Verification items for this drawing (mm, ordinates from the low corner). A direction names the side the tool comes from. Round coordinates to 2 decimals unless told otherwise and drop trailing zeros. Loops run counter-clockwise (first coordinate to the right, second up) from the corner with the lowest first, then second, coordinate; pieces in that order, holes last. Notation, with made-up numbers: M 73,-24 L 87,-24 A21 ccw 87,-20 Z; hole C 41.25,30.25 d10. An arc over 180 degrees is marked long. One line per item, written item: value.
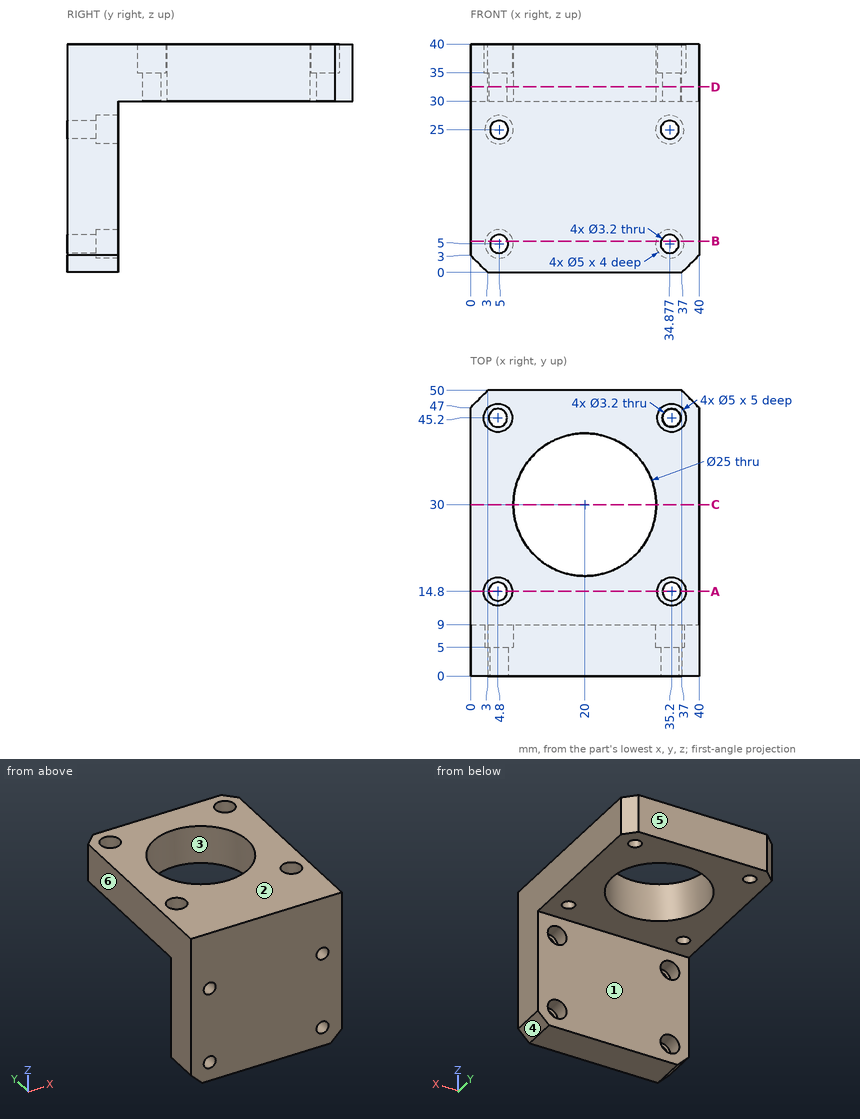
(1) Tool access check on the marked faces 1 and 2. Record the directions out of +Z, -Z, +X, -X, +Y, -Y that give a thin tool (end or side, any length) a straight path to the whole face; none if there is none.
Completed:
face 1: -Z, +X, -X, +Y
face 2: +Z, +X, -X, +Y, -Y
(2) Mould release check, pull along X, two halves, no side actions. Record for the marked faces 3, 4, 5 and 6: +X half, -X half, draft (parallel to the pull), parting line (faces both ways), or undercut.
Completed:
face 3: undercut
face 4: +X half
face 5: draft
face 6: -X half
(3) Sectioned sample at A-A on y = 14.8. Enter the section's corners in (x, z).
Completed:
outline: M 0,30 L 3.2,30 L 3.2,35 L 2.3,35 L 2.3,40 L 0,40 Z; M 6.4,30 L 33.6,30 L 33.6,35 L 32.7,35 L 32.7,40 L 7.3,40 L 7.3,35 L 6.4,35 Z; M 36.8,30 L 40,30 L 40,40 L 37.7,40 L 37.7,35 L 36.8,35 Z
(4) Depth check by flat-ended pin: pin 1 Ø2.5 at (x, z) = (34, 5.5) entering from +Y; pin 2 Ø6 at (x, y) = (33.5, 44) entering from -Z; pin 3 Ø1.9 at (x, y) = (35.2, 45.2) entering from +Z; pin 4 Ø6.5 at (x, z) = (34.88, 5) entering from +Y. Enter the tip coordinate at first touch or a pass-through.
Completed:
pin 1: stops at y = 5
pin 2: stops at z = 30
pin 3: passes through
pin 4: stops at y = 9
(5) Sectioned sample at D-D on z = 32.5. Enter the section's corners in (x, y), and give its area (3 significant figures).
Completed:
outline: M 0,0 L 40,0 L 40,47 L 37,50 L 3,50 L 0,47 Z; hole C 4.8,14.8 d3.2; hole C 4.8,45.2 d3.2; hole C 20,30 d25; hole C 35.2,14.8 d3.2; hole C 35.2,45.2 d3.2
area: 1,470 mm^2
(6) Sectioned sample at B-B on z = 5.5. Enter the section's corners in (x, y).
Completed:
outline: M 0,0 L 3.48,0 L 3.48,5 L 2.55,5 L 2.55,9 L 0,9 Z; M 6.52,0 L 33.36,0 L 33.36,5 L 32.43,5 L 32.43,9 L 7.45,9 L 7.45,5 L 6.52,5 Z; M 36.4,0 L 40,0 L 40,9 L 37.33,9 L 37.33,5 L 36.4,5 Z
(7) Thickness scan on L1, parallel to Y at x = 35, z = 37; L2, parallel to Y at x = 35, z = 33; L3, parallel to X at y = 6, z = 5. Record the ranges inside material, lowest first. Write a range as from..to.
Completed:
L1: y = 0..12.31, 17.29..42.71, 47.69..50
L2: y = 0..13.21, 16.39..43.61, 46.79..50
L3: x = 0..2.5, 7.5..32.38, 37.38..40
(8) Sectioned sample at C-C on y = 30. Enter the section's corners in (x, z).
Completed:
outline: M 0,30 L 7.5,30 L 7.5,40 L 0,40 Z; M 32.5,30 L 40,30 L 40,40 L 32.5,40 Z
